```python
from build123d import *

# Parameters (mm, degrees)
F0_W     = 36.736786
F0_H     = 41.465297
F1_DEPTH = 500
F2_R     = 5
F3_T     = -3


with BuildPart() as f1:
    # F0 (on Front) → F1 (new body)
    with BuildSketch(Plane.XZ):
        with Locations((18.368393, 20.732648)):
            Rectangle(F0_W, F0_H)
    extrude(amount=F1_DEPTH)

    # F2
    f2_edges = [f1.edges().sort_by_distance(p)[0] for p in [
        (36.736786, -250, 41.465297),
        (0, -250, 41.465297),
        (36.736786, -250, 0),
        (0, -250, 0),
    ]]
    fillet(f2_edges, radius=F2_R)

    # F3
    f3_openings = [f1.faces().sort_by_distance(p)[0] for p in [
        (18.368393, -500, 20.732649),
        (18.368393, 0, 20.732649),
    ]]
    offset(amount=F3_T, openings=f3_openings)


solid = f1.part
```
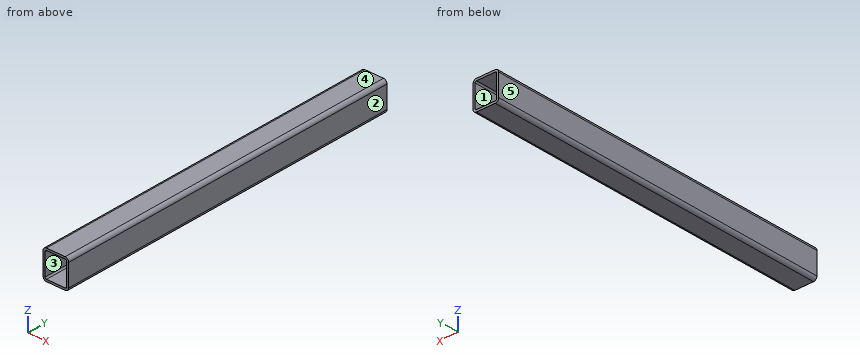
Design review of the part built by this model. Coordinates are the model's own, in mm. Face numbers are marked on the shaded views. A direction names the side the tool comes from. Round coordinates to 2 decimals unless told otherwise and drop trailing zeros. Order: outer loops, then holes, each group sorted by start corner. A loop starts at its lowest first (then second) coordinate and runs counter-clockwise, first axis right, second up. Notation, with made-up numbers: M 69.25,18.25 L 114.25,18.25 A4 ccw 114.25,22.25 Z; hole C 30,72 d9. An arc over 180 degrees is marked long. Put each result on its own line as item: value.
Q1. Consider section A-A (z = 13.5). State the section outline as (x, y) points.
Reported:
outline: M 0,-500 L 3,-500 L 3,0 L 0,0 Z; M 33.74,-500 L 36.74,-500 L 36.74,0 L 33.74,0 Z
Q2. Machinability: for the marked faces 1 and 2, which of the approach directions +Z, -Z, +X, -X, +Y, -Y give a long, thin tool a straight path to every point of the face, cutting with its end or side? Answer none if there is none.
Reported:
face 1: +Y, -Y
face 2: +Z, -Z, +X, +Y, -Y
Q3. Draft analysis for pull direction X (two halves, no side actions). For the marked faces 3, 4 and 5, state which applies: released by +X, released by -X, zero draft, split by the parting line, or undercut.
Reported:
face 3: undercut
face 4: zero draft
face 5: released by -X
Q4. Consider section B-B (x = 24). State the section outline as (y, z) points, and give its area (3 significant figures).
Reported:
outline: M -500,0 L 0,0 L 0,3 L -500,3 Z; M -500,38.47 L 0,38.47 L 0,41.47 L -500,41.47 Z
area: 3,000 mm²
Q5. To check wall thickness, follow line 1 (X direction, y = -155.5, z = 30); line 2 (Z direction, x = 26, y = -479.5); line 3 (X direction, y = -365, z = 37). State the ranges of each line that lie inside material, in increasing order.
Reported:
line 1: 0 to 3, 33.74 to 36.74
line 2: 0 to 3, 38.47 to 41.47
line 3: 0.03 to 3.07, 33.66 to 36.71
Q6. Consider section C-C (y = -157.5). State the section outline as (x, z) points.
Reported:
outline: M 0,5 A5 ccw 5,0 L 31.74,0 A5 ccw 36.74,5 L 36.74,36.47 A5 ccw 31.74,41.47 L 5,41.47 A5 ccw 0,36.47 Z; hole M 3,5 A2 ccw 5,3 L 31.74,3 A2 ccw 33.74,5 L 33.74,36.47 A2 ccw 31.74,38.47 L 5,38.47 A2 ccw 3,36.47 Z
